```python
from build123d import *

# Parameters (mm, degrees)
F0_R     = 1.5875
F0_R_2   = 2.0193
F0_R_3   = 3.175
F0_W     = 77.089
F0_H     = 6.35
F0_R_4   = 2.413
F1_DEPTH = 5.842
F2_R     = 9.525
F3_R     = 5.08


with BuildPart() as f1:
    # F0 (on Front) → F1 (new body)
    with BuildSketch(Plane.XZ):
        Polygon((12.7, 12.7), (-12.7, 12.7), (-12.7, 3.175), (-12.7, -3.175), (-12.7, -12.7), (12.7, -12.7), align=None)
        with Locations((0, -10.16)):
            Circle(F0_R, mode=Mode.SUBTRACT)
        with Locations((-9.271, 0)):
            Circle(F0_R_2, mode=Mode.SUBTRACT)
        Circle(F0_R_3, mode=Mode.SUBTRACT)
        with Locations((9.271, 0)):
            Circle(F0_R_2, mode=Mode.SUBTRACT)
        with Locations((0, 10.16)):
            Circle(F0_R, mode=Mode.SUBTRACT)
        with Locations((-51.2445, 0)):
            Rectangle(F0_W, F0_H)
        Polygon((-89.789, -3.175), (-89.789, 3.175), (-89.789, 12.7), (-115.189, 12.7), (-115.189, -12.7), (-89.789, -12.7), align=None)
        with Locations((-110.363, -7.874)):
            Circle(F0_R_4, mode=Mode.SUBTRACT)
        with Locations((-94.615, -7.874)):
            Circle(F0_R_4, mode=Mode.SUBTRACT)
        with Locations((-110.363, 7.874)):
            Circle(F0_R_4, mode=Mode.SUBTRACT)
        with Locations((-94.615, 7.874)):
            Circle(F0_R_4, mode=Mode.SUBTRACT)
    extrude(amount=F1_DEPTH)

    # F2
    f2_edges = [f1.edges().sort_by_distance(p)[0] for p in [
        (12.7, -2.921, 12.7),
        (12.7, -2.921, -12.7),
    ]]
    fillet(f2_edges, radius=F2_R)

    # F3
    f3_edges = [f1.edges().sort_by_distance(p)[0] for p in [
        (-12.7, -2.921, -12.7),
        (-12.7, -2.921, 12.7),
    ]]
    fillet(f3_edges, radius=F3_R)


solid = f1.part
```
For this review, take the finished solid that the model builds, in its own axes (mm). A direction names the side the tool comes from. Round coordinates to 2 decimals unless told otherwise and drop trailing zeros. Write each loop counter-clockwise with the first axis right and the second up, starting at its lowest first coordinate (ties: lowest second). Pieces come first, ordered by that corner, then holes. Notation, with made-up numbers: (9.5, 69.5) - (24.5, 69.5) arc R13 ccw to (24.5, 89.5) - close; hole circle Ø11 at (1.25, 87). An arc over 180 degrees is marked (long way). Use CSV: the item, a comma, the result in double quotes.
1) Clearance check with a flat-ended pin moving along its axis: pin 1 Ø1.8 at (x, y) = (-39, -3) entering from +Z (3 decimals). State where the tip first meets the part, or that it passes through.
Conclusion:
pin 1,"stops at z = 3.175"
2) For faces 1 (the cylindrical face through (9.84, -2.96, 9.98)), 2 (the flat face through (-12.7, -3, 5)), 3 (the cylindrical face through (-11.172, -2.962, -11.251)), list the 3-axis set-ups (+Z, -Z, +X, -X, +Y, -Y) from which the entire face can be reached by the end or side of a thin tool; tool diameter is ignored.
Conclusion:
face 1,"+Z, +X, +Y, -Y"
face 2,"+Z, +Y, -Y"
face 3,"-Z, +Y, -Y"
3) Add section B-B on z = 0. Write out the cut boundary in (x, y) (3 decimals).
Conclusion:
outline,"(-115.189, -5.842) - (-11.29, -5.842) - (-11.29, 0) - (-115.189, 0) - close; (-7.252, -5.842) - (-3.175, -5.842) - (-3.175, 0) - (-7.252, 0) - close; (3.175, -5.842) - (7.252, -5.842) - (7.252, 0) - (3.175, 0) - close; (11.29, -5.842) - (12.7, -5.842) - (12.7, 0) - (11.29, 0) - close"
4) Add section D-D on x = -76. Write out the cut boundary in (y, z) (3 decimals).
Conclusion:
outline,"(-5.842, -3.175) - (0, -3.175) - (0, 3.175) - (-5.842, 3.175) - close"
5) The part is to be moulded in two halves that separate along X. For faces 4 (the flat face through (-2, -3, -12.7)), 5 (the flat face through (12.7, -3, 0)), 6 (the cylindrical face through (-11.172, -2.962, 11.251)), 7 (the flat face through (-52, -3, -3.175)), say which applies: pulls with the +X half, pulls with the -X half, needs draft (parallel to the pull), parting line crosses it, or undercut.
Conclusion:
face 4,"needs draft"
face 5,"pulls with the +X half"
face 6,"undercut"
face 7,"undercut"
6) Add section A-A on x = 0. Write out the cut boundary in (y, z) (1 decimal), and give its area (3 significant figures).
Conclusion:
outline,"(-5.8, -12.7) - (0, -12.7) - (0, -11.7) - (-5.8, -11.7) - close; (-5.8, -8.6) - (0, -8.6) - (0, -3.2) - (-5.8, -3.2) - close; (-5.8, 3.2) - (0, 3.2) - (0, 8.6) - (-5.8, 8.6) - close; (-5.8, 11.7) - (0, 11.7) - (0, 12.7) - (-5.8, 12.7) - close"
area,"74.2 mm^2"
7) Add section C-C on y = -3.5. Count the separate pieces of the cut face and the enclosed holes in it, and give its area (3 significant figures).
Conclusion:
separate pieces,"1"
enclosed holes,"9"
area,"1,580 mm^2"
8) Wall thickness on line 1 along Z through (x, y) = (0, -2.15) (1 decimal); line 2 along X through (y, z) = (-0.95, 3.75); line 3 along X through (y, z) = (-3.6, 2.75): over which ranges is each line inside the solid? List them lowest first. Write a range as from..to.
Conclusion:
line 1,"z = -12.7..-11.7, -8.6..-3.2, 3.2..8.6, 11.7..12.7"
line 2,"x = -115.19..-89.79, -12.7..12.68"
line 3,"x = -115.19..-1.59, 1.59..12.7"
